from build123d import *

# Parameters (mm, degrees)
CROQUIS1_W              = 50
CROQUIS1_H              = 30
SALIENTE_EXTRUIR1_DEPTH = 20
CORTAR_EXTRUIR1_DEPTH   = 1
CROQUIS3_W              = 31.537351035
CROQUIS3_H              = 3.738113103
SALIENTE_EXTRUIR2_DEPTH = 50
CROQUIS4_W              = 19.19980798
CROQUIS4_H              = 3.778383676
SALIENTE_EXTRUIR3_DEPTH = 10


with BuildPart() as part:
    # Croquis1 → Saliente-Extruir1 (new body)
    with BuildSketch(Plane(origin=(0, 0, 0), x_dir=(1, 0, 0), z_dir=(0, 1, 0))):
        Rectangle(CROQUIS1_W, CROQUIS1_H)
    extrude(amount=SALIENTE_EXTRUIR1_DEPTH)

    # Croquis2 → Cortar-Extruir1 (cut)
    with BuildSketch(Plane(origin=(0, 20, 0), x_dir=(1, 0, 0), z_dir=(0, 1, 0))):
        with BuildLine():
            Line((-17.950861779, 10.424113245), (-6.810393923, 10.424113245))
            ThreePointArc((-6.810393923, 10.424113245), (-5.547045664, 9.900817262), (-5.023749681, 8.637469002))
            Line((-5.023749681, 8.637469002), (-5.023749681, -7.293911131))
            ThreePointArc((-5.023749681, -7.293911131), (-5.541364738, -8.543544422), (-6.790998029, -9.061159479))
            Line((-6.790998029, -9.061159479), (-18.510223917, -9.061159479))
            ThreePointArc((-18.510223917, -9.061159479), (-19.415274859, -7.898406759), (-19.737506021, -6.460603513))
            Line((-19.737506021, -6.460603513), (-19.737506021, 8.637469002))
            ThreePointArc((-19.737506021, 8.637469002), (-19.214210038, 9.900817262), (-17.950861779, 10.424113245))
        make_face()
    extrude(amount=-CORTAR_EXTRUIR1_DEPTH, mode=Mode.SUBTRACT)

    # Croquis3 → Saliente-Extruir2 (add)
    with BuildSketch(Plane.XZ):
        with Locations((-0.297550373, 13.130943449)):
            Rectangle(CROQUIS3_W, CROQUIS3_H)
    extrude(amount=SALIENTE_EXTRUIR2_DEPTH)

    # Croquis4 → Saliente-Extruir3 (add)
    with BuildSketch(Plane.XY.offset(15)):
        with Locations((-0.62783913, -1.889191838)):
            Rectangle(CROQUIS4_W, CROQUIS4_H)
    extrude(amount=SALIENTE_EXTRUIR3_DEPTH)


solid = part.part
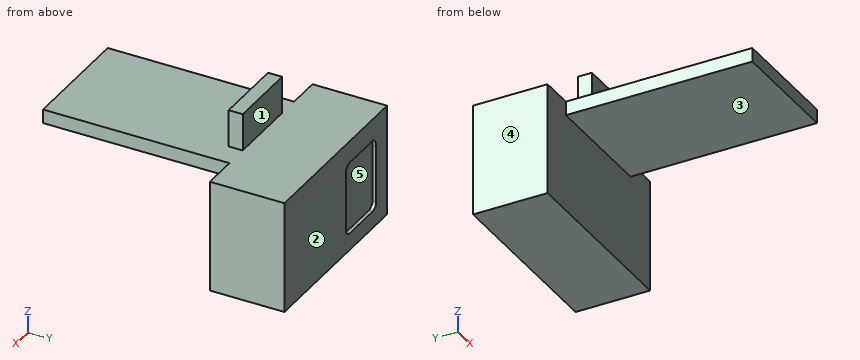
Check sheet for the modelled part. Datum: model origin and axes. Units: mm. Face numbers are marked on the shaded views. A direction names the side the tool comes from. Round coordinates to 2 decimals unless told otherwise and drop trailing zeros. Order: outer loops, then holes, each group sorted by start corner. A loop starts at its lowest first (then second) coordinate and runs counter-clockwise, first axis right, second up.
Q1. Cross-section at C-C, the plane z = -5.5. Enter the section's corners in (x, y).
Filled sheet:
outline: (-25, 0) - (25, 0) - (25, 20) - (-5.02, 20) - (-5.02, 19) - (-19.74, 19) - (-19.74, 20) - (-25, 20) - close
Q2. Draft check along X on the marked faces 3, 4 and 5. Enter one of: pulls with the +X half, pulls with the -X half, needs draft (parallel to the pull), parting line crosses it, or undercut.
Filled sheet:
face 3: needs draft
face 4: pulls with the -X half
face 5: undercut
Q3. Cross-section at D-D, the plane x = 21. Enter the section's corners in (y, z), plus the area to 3 significant figures.
Filled sheet:
outline: (0, -15) - (20, -15) - (20, 15) - (0, 15) - close
area: 600 mm2
Q4. Depth check by flat-ended pin: P1, Ø1.5, axis at y = -33.5, z = 13.5, coming from the +X side; P2, Ø15, axis at x = -5.5, z = -2.5, coming from the -Y side; P3, Ø16, axis at x = -15.5, z = -4.5, coming from the +Y side; P4, Ø1, axis at x = 16, y = 8.5, coming from the +Z side. Enter the tip coordinate at first touch or a pass-through.
Filled sheet:
P1: stops at x = 15.47
P2: stops at y = 0
P3: stops at y = 20
P4: stops at z = 15
Q5. Scan lines: L1, parallel to Z at x = 2, y = -30; L2, parallel to Y at x = 11, z = 6.5; L3, parallel to Z at x = 22, y = 10.5. Record each from-to range of solid material in increasing order.
Filled sheet:
L1: z = 11.26 to 15
L2: y = 0 to 20
L3: z = -15 to 15
Q6. Cross-section at B-B, the plane x = 1.5. Enter the section's corners in (y, z).
Filled sheet:
outline: (-50, 11.26) - (0, 11.26) - (0, -15) - (20, -15) - (20, 15) - (0, 15) - (0, 25) - (-3.78, 25) - (-3.78, 15) - (-50, 15) - close
Q7. Cross-section at A-A, the plane y = -2. Enter the section's corners in (x, z).
Filled sheet:
outline: (-16.07, 11.26) - (15.47, 11.26) - (15.47, 15) - (8.97, 15) - (8.97, 25) - (-10.23, 25) - (-10.23, 15) - (-16.07, 15) - close
Q8. Set-up check for the marked faces 1 and 2: record each of +Z, -Z, +X, -X, +Y, -Y from which the full face is reachable in a straight line by a thin tool's end or side.
Filled sheet:
face 1: +Z, +X, -X, +Y
face 2: +Z, -Z, +X, -X, +Y
